Geometry: final body of the model. Coordinates: model frame, mm. A direction names the side the tool comes from. Give positions to 0.01 mm unless a question says otherwise; leave off trailing zeros. Write each loop counter-clockwise with the first axis right and the second up, starting at its lowest first coordinate (ties: lowest second). Pieces come first, ordered by that corner, then holes.
Q1. Section C-C (y = 50.5). Return the cut outline in (x, z).
Q2. Section B-B (y = 65). Return the cut outline in (x, z).
Q3. Section A-A (x = 11.43). Return the cut outline in (y, z).
Q4. Section D-D (x = 72). Return the cut outline in (y, z).
Q5. Mould query, pull axis X, two halves, no side actions, for faces 1 (the cylindrical face through (11.35, 41.91, 3.22)), 2 (the flat face through (0, 57, 3)), 3 (the cylindrical face through (11.179, 91.437, 3.131)). Classes: +X half, -X half, draft (parallel to the pull), parting line (faces both ways), or undercut.
Q6. Line query: line 1 (X direction, y = 59.5, z = 3.5); line 2 (X direction, y = 46.5, z = 4); line 3 (Y direction, x = 63.5, z = 11). Output: solid intervals per line, ascending.
Q7. Reachability of faces 4 (the flat face through (91.44, 46, 6)), 5 (the flat face through (57, 57.15, 6)), 6 (the flat face through (15.24, 63, 3)), 7 (the flat face through (16, 63, 6.35)), 8 (the flat face through (46, 34.29, 6)) from +Z, -Z, +X, -X, +Y, -Y: full face, straight path, thin tool, end or side. Return the list, or none.
Q8. Pin query (flat end, axial travel): pin 1 Ø11.5 at (x, y) = (16, 58.5) entering from +Z; pin 2 Ø5 at (y, z) = (71, 4) entering from +X. Return the tip coordinate at first contact, or that it passes through.
Autodesk Inventor part; units mm, degrees
ref_plane "YZ Plane" through (0, 0, 0) normal (1, 0, 0) x (0, 1, 0)
ref_plane "XZ Plane" through (0, 0, 0) normal (0, 1, 0) x (-1, 0, 0)
ref_plane "XY Plane" through (0, 0, 0) normal (0, 0, 1) x (1, 0, 0)
sketch "Sketch1" plane through (0, 0, 0) normal (0, 0, 1) x (1, 0, 0)
  line L0 (0, 0) -> (22.86, 0)
  line L1 (22.86, 0) -> (22.86, 91.44)
  line L2 (22.86, 91.44) -> (0, 91.44)
  line L3 (0, 91.44) -> (0, 0)
  line L4 (22.86, 57.15) -> (91.44, 57.15)
  line L5 (91.44, 57.15) -> (91.44, 34.29)
  line L6 (91.44, 34.29) -> (22.86, 34.29)
  line L7 (22.86, 34.29) -> (22.86, 57.15)
  line L8 (11.43, 80.01) -> (11.43, 11.43) construction
  line L9 (7.62, 80.01) -> (7.62, 11.43)
  line L10 (15.24, 11.43) -> (15.24, 80.01)
  arc A0 (15.24, 80.01) -> (7.62, 80.01) centre (11.43, 80.01) ccw
  arc A1 (7.62, 11.43) -> (15.24, 11.43) centre (11.43, 11.43) ccw
  arc A2 (22.86, 80.01) -> (0, 80.01) centre (11.43, 80.01) ccw
  arc A3 (0, 11.43) -> (22.86, 11.43) centre (11.43, 11.43) ccw
  point P0 (11.43, 45.72)
  point P1 (-17.5605, -7.6237)
  dimension "d0" = 22.86
  dimension "d1" = 91.44
  dimension "d2" = 68.58
  dimension "d3" = 22.86
  dimension "d4" = 34.29
  dimension "d5" = 68.58
  dimension "d6" = 7.62
  dimension "d7" = 11.43
  dimension "d8" = 11.43
  dimension "d9" = 0
  dimension "d10" = 0
extrude "Extrusion1" add sketch "Sketch1" along normal blind 12.7 contours A3 L3 A2 L1 | L1 L4 L5 L6
sketch "Sketch2" plane through (0, 0, 12.7) normal (0, 0, 1) x (1, 0, 0)
  line L0 (22.86, 0) -> (0, 0)
  line L1 (0, 0) -> (0, 91.44)
  line L2 (0, 91.44) -> (22.86, 91.44)
  line L3 (22.86, 91.44) -> (22.86, 0)
  line L4 (0, 80.01) -> (0, 11.43)
  line L5 (22.86, 57.15) -> (22.86, 80.01)
  arc A0 (22.86, 80.01) -> (0, 80.01) centre (11.43, 80.01) ccw
  arc A1 (0, 11.43) -> (22.86, 11.43) centre (11.43, 11.43) ccw
  point P0 (0, 0)
  point P1 (0, 11.43)
  dimension "d13" = 0
  dimension "d14" = 0
extrude "Extrusion2" cut sketch "Sketch2" against normal blind 6.35 contours A1 L1 A0 L3
sketch "Sketch3" plane through (0, 0, 6.35) normal (0, 0, 1) x (1, 0, 0)
  line L0 (22.86, 34.29) -> (91.44, 34.29)
  line L1 (22.86, 34.29) -> (0, 34.29)
  line L2 (0, 34.29) -> (0, 0)
  line L3 (0, 0) -> (22.86, 0)
  line L4 (22.86, 0) -> (22.86, 34.29)
  line L5 (0, 11.43) -> (0, 80.01)
  arc A0 (0, 11.43) -> (22.86, 11.43) centre (11.43, 11.43) ccw
  point P0 (0, 0)
  dimension "d17" = 0
extrude "Extrusion3" cut sketch "Sketch3" against normal blind 107.95 contours L4 A0 L2 L1
sketch "Sketch4" plane through (0, 0, 6.35) normal (0, 0, 1) x (1, 0, 0)
  line L0 (22.86, 34.29) -> (0, 34.29)
  line L1 (0, 34.29) -> (0, 41.91)
  line L2 (22.86, 41.91) -> (22.86, 34.29)
  arc A0 (7.62, 45.72) -> (15.24, 45.72) centre (11.43, 45.72) ccw
  line L3 (15.24, 34.29) -> (15.24, 80.01)
  line L4 (15.24, 41.91) -> (15.24, 45.72)
  line L5 (7.62, 80.01) -> (7.62, 34.29)
  line L6 (7.62, 41.91) -> (7.62, 45.72)
  line L7 (0, 41.91) -> (7.62, 41.91)
  line L8 (15.24, 41.91) -> (22.86, 41.91)
  point P0 (0, 0)
  dimension "d20" = 22.86
  dimension "d21" = 7.62
  dimension "d22" = 7.62
extrude "Extrusion4" add sketch "Sketch4" against normal blind 6.35 contours L0 L5 A0 L3
properties part number "Slider2"
Computed:
1. outline: (0, 0) - (7.62, 0) - (7.62, 6.35) - (0, 6.35) - close; (15.24, 0) - (91.44, 0) - (91.44, 12.7) - (22.86, 12.7) - (22.86, 6.35) - (15.24, 6.35) - close
2. outline: (0, 0) - (7.62, 0) - (7.62, 6.35) - (0, 6.35) - close; (15.24, 0) - (22.86, 0) - (22.86, 6.35) - (15.24, 6.35) - close
3. outline: (34.29, 0) - (41.91, 0) - (41.91, 6.35) - (34.29, 6.35) - close; (83.82, 0) - (91.44, 0) - (91.44, 6.35) - (83.82, 6.35) - close
4. outline: (34.29, 0) - (57.15, 0) - (57.15, 12.7) - (34.29, 12.7) - close
5. face 1: undercut
5. face 2: -X half
5. face 3: parting line
6. line 1: x = 0 to 7.62, 15.24 to 22.86
6. line 2: x = 0 to 7.62, 15.24 to 91.44
6. line 3: y = 34.29 to 57.15
7. face 4: +Z, -Z, +X, +Y, -Y
7. face 5: +Z, -Z, +X, +Y
7. face 6: +Z, -Z
7. face 7: +Z, -X, +Y, -Y
7. face 8: +Z, -Z, +X, -X, -Y
8. pin 1: stops at z = 6.35
8. pin 2: stops at x = 22.86
